```python
from build123d import *

# Parameters (mm, degrees)
SKETCH1_W             = 40
SKETCH1_H             = 40
CROSS_JOINER_DEPTH    = 3
BOLT_HOLES_DEPTH      = 29.442925307
BOLT_HOLES_DEPTH_BACK = 29.442925307
SKETCH2_R             = 1.7


with BuildPart() as part:
    # Sketch1 → Cross Joiner (new body)
    with BuildSketch(Plane(origin=(0, 0, 0), x_dir=(1, 0, 0), z_dir=(0, 1, 0))):
        Rectangle(SKETCH1_W, SKETCH1_H)
    extrude(amount=CROSS_JOINER_DEPTH)

    # Sketch2 → Bolt Holes (cut, two sides: drawn at the far end of the back side and taken through both)
    with BuildSketch(Plane(origin=(0, 0, 0), x_dir=(1, 0, 0), z_dir=(0, 1, 0)).offset(-BOLT_HOLES_DEPTH_BACK)):
        with Locations(Location((-12, -12, 0), (0, 0, 270))):
            Circle(SKETCH2_R)
        with Locations(Location((-12, 12, 0), (0, 0, 270))):
            Circle(SKETCH2_R)
        with Locations(Location((12, -12, 0), (0, 0, 270))):
            Circle(SKETCH2_R)
        with Locations(Location((12, 12, 0), (0, 0, 270))):
            Circle(SKETCH2_R)
    extrude(amount=BOLT_HOLES_DEPTH + BOLT_HOLES_DEPTH_BACK, mode=Mode.SUBTRACT)


solid = part.part
```
Check sheet for the modelled part. Datum: model origin and axes. Units: mm. Give positions to 0.01 mm unless a question says otherwise; leave off trailing zeros. Order: outer loops, then holes, each group sorted by start corner. A loop starts at its lowest first (then second) coordinate and runs counter-clockwise, first axis right, second up. Notation, with made-up numbers: (51, -3) -> (82, -3) arc R11 cw to (82, 16) -> close; hole circle Ø3 at (-12.5, 23). An arc over 180 degrees is marked (long way). Return JSON: item names as keys, results as strings.
1. Cross-section at B-B, the plane y = 1.6. Record the cut outline in (x, z).
From the geometry:
{"outline": "(-20, -20) -> (20, -20) -> (20, 20) -> (-20, 20) -> close; hole circle Ø3.4 at (-12, -12); hole circle Ø3.4 at (-12, 12); hole circle Ø3.4 at (12, -12); hole circle Ø3.4 at (12, 12)"}
2. Mould release check, pull along X, two halves, no side actions. Record for faces 1 (the cylindrical face through (12.51, 1.48, 13.62)), 2 (the flat face through (20, 1, 0)), 3 (the cylindrical face through (-12.65, 1.48, 13.57)), 4 (the flat face through (0, 3, 0)): +X half, -X half, draft (parallel to the pull), parting line (faces both ways), or undercut.
From the geometry:
{"face 1": "undercut", "face 2": "+X half", "face 3": "undercut", "face 4": "draft"}
3. Cross-section at A-A, the plane z = -12. Record the cut outline in (x, y).
From the geometry:
{"outline": "(-20, 0) -> (-13.7, 0) -> (-13.7, 3) -> (-20, 3) -> close; (-10.3, 0) -> (10.3, 0) -> (10.3, 3) -> (-10.3, 3) -> close; (13.7, 0) -> (20, 0) -> (20, 3) -> (13.7, 3) -> close"}
4. Cross-section at C-C, the plane x = -12. Record the cut outline in (y, z), plus the area to 3 significant figures.
From the geometry:
{"outline": "(0, -20) -> (3, -20) -> (3, -13.7) -> (0, -13.7) -> close; (0, -10.3) -> (3, -10.3) -> (3, 10.3) -> (0, 10.3) -> close; (0, 13.7) -> (3, 13.7) -> (3, 20) -> (0, 20) -> close", "area": "99.6 mm^2"}
5. Go/stop test with a flat-tipped pin: P1, Ø3, axis at x = -12, z = -12, coming from the -Y side. Record where the tip stops, or that it passes through.
From the geometry:
{"P1": "through"}
6. Material ranges on probe 1 along X at (y, z) = (1.3, 12); probe 2 along X at (y, z) = (1.4, 13), recorded low to high. Write a range as [from, to].
From the geometry:
{"probe 1": "[-20, -13.7], [-10.3, 10.3], [13.7, 20]", "probe 2": "[-20, -13.37], [-10.63, 10.63], [13.37, 20]"}
